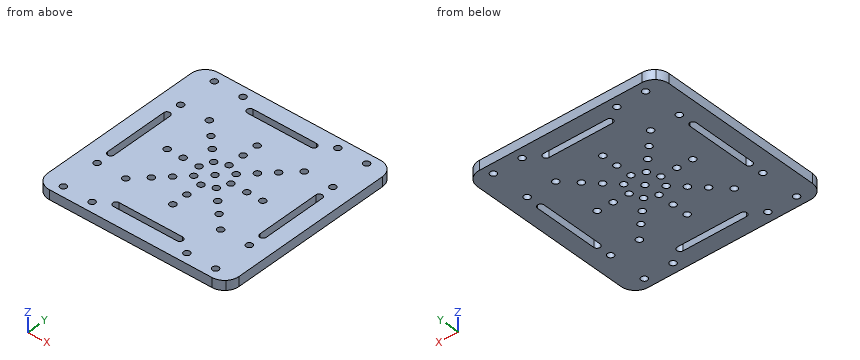
from build123d import *

# Parameters (mm, degrees)
F0_W     = 120
F0_H     = 6
F1_DEPTH = 120
F3_D     = 4
F3_DEPTH = 8
F3_TIP   = 1.2017212381
F4_DEPTH = 8
F5_DEPTH = 6


with BuildPart() as f1:
    # F0 (on Front) → F1 (new body)
    with BuildSketch(Plane.XZ):
        with Locations((60, 3)):
            Rectangle(F0_W, F0_H)
    extrude(amount=F1_DEPTH)

    # F3
    with Locations(Plane(origin=(0, 0, 0), x_dir=(1, 0, 0), z_dir=(0, 0, -1))):
        with Locations((12.2512626585, 113.7487373415), (12.2512626585, 89.7487373415), (30.2512626585, 89.7487373415), (30.2512626585, 113.7487373415), (89.7487373415, 113.7487373415), (89.7487373415, 89.7487373415), (107.7487373415, 89.7487373415), (107.7487373415, 113.7487373415), (107.7487373415, 30.2512626585), (89.7487373415, 30.2512626585), (89.7487373415, 6.2512626585), (107.7487373415, 6.2512626585), (30.2512626585, 6.2512626585), (12.2512626585, 30.2512626585), (30.2512626585, 30.2512626585), (12.2512626585, 6.2512626585), (38.7867965644, 38.7867965644), (45.8578643763, 45.8578643763), (30, 60), (40, 60), (45.8578643763, 74.1421356237), (38.7867965644, 81.2132034356), (60, 80), (60, 90), (81.2132034356, 81.2132034356), (74.1421356237, 74.1421356237), (80, 60), (90, 60), (81.2132034356, 38.7867965644), (74.1421356237, 45.8578643763), (60, 40), (60, 30), (52.9289321881, 67.0710678119), (60, 60), (50, 60), (52.9289321881, 52.9289321881), (60, 50), (67.0710678119, 52.9289321881), (70, 60), (67.0710678119, 67.0710678119), (60, 70)):
            Hole(F3_D / 2, depth=F3_DEPTH)
            with Locations((0, 0, -(F3_DEPTH + F3_TIP / 2))):  # 118° drill point
                Cone(0, F3_D / 2, F3_TIP, mode=Mode.SUBTRACT)

    # F2 (on Top) → F4 (cut)
    with BuildSketch(Plane.XY):
        with BuildLine():
            Line((10.2512626585, -40), (10.2512626585, -60))
            Line((10.2512626585, -60), (14.2512626585, -60))
            Line((14.2512626585, -60), (14.2512626585, -40))
            ThreePointArc((14.2512626585, -40), (12.2512626585, -38), (10.2512626585, -40))
        make_face()
        with BuildLine():
            Line((14.2512626585, -60), (10.2512626585, -60))
            Line((10.2512626585, -60), (10.2512626585, -80))
            ThreePointArc((10.2512626585, -80), (12.2512626585, -82), (14.2512626585, -80))
            Line((14.2512626585, -80), (14.2512626585, -60))
        make_face()
        with BuildLine():
            Line((60, -109.7487373415), (60, -105.7487373415))
            Line((60, -105.7487373415), (40, -105.7487373415))
            ThreePointArc((40, -105.7487373415), (38, -107.7487373415), (40, -109.7487373415))
            Line((40, -109.7487373415), (60, -109.7487373415))
        make_face()
        with BuildLine():
            Line((80, -105.7487373415), (60, -105.7487373415))
            Line((60, -105.7487373415), (60, -109.7487373415))
            Line((60, -109.7487373415), (80, -109.7487373415))
            ThreePointArc((80, -109.7487373415), (82, -107.7487373415), (80, -105.7487373415))
        make_face()
        with BuildLine():
            Line((105.7487373415, -40), (105.7487373415, -60))
            Line((105.7487373415, -60), (109.7487373415, -60))
            Line((109.7487373415, -60), (109.7487373415, -40))
            ThreePointArc((109.7487373415, -40), (107.7487373415, -38), (105.7487373415, -40))
        make_face()
        with BuildLine():
            Line((109.7487373415, -60), (105.7487373415, -60))
            Line((105.7487373415, -60), (105.7487373415, -80))
            ThreePointArc((105.7487373415, -80), (107.7487373415, -82), (109.7487373415, -80))
            Line((109.7487373415, -80), (109.7487373415, -60))
        make_face()
        with BuildLine():
            Line((40, -14.2512626585), (60, -14.2512626585))
            Line((60, -14.2512626585), (60, -10.2512626585))
            Line((60, -10.2512626585), (40, -10.2512626585))
            ThreePointArc((40, -10.2512626585), (38, -12.2512626585), (40, -14.2512626585))
        make_face()
        with BuildLine():
            Line((60, -10.2512626585), (60, -14.2512626585))
            Line((60, -14.2512626585), (80, -14.2512626585))
            ThreePointArc((80, -14.2512626585), (82, -12.2512626585), (80, -10.2512626585))
            Line((80, -10.2512626585), (60, -10.2512626585))
        make_face()
    extrude(amount=F4_DEPTH, mode=Mode.SUBTRACT)

    # F2 (on Top) → F5 (cut)
    with BuildSketch(Plane.XY):
        with BuildLine():
            Line((120, -120), (120, -111))
            ThreePointArc((120, -111), (119.3149157926, -114.4441508913), (117.3639610307, -117.3639610307))
            Line((117.3639610307, -117.3639610307), (120, -120))
        make_face()
        with BuildLine():
            ThreePointArc((117.3639610307, -117.3639610307), (114.4441508913, -119.3149157926), (111, -120))
            Line((111, -120), (120, -120))
            Line((120, -120), (117.3639610307, -117.3639610307))
        make_face()
        with BuildLine():
            Line((2.6360389693, -117.3639610307), (0, -120))
            Line((0, -120), (9, -120))
            ThreePointArc((9, -120), (5.5558491087, -119.3149157926), (2.6360389693, -117.3639610307))
        make_face()
        with BuildLine():
            ThreePointArc((2.6360389693, -117.3639610307), (0.6850842074, -114.4441508913), (0, -111))
            Line((0, -111), (0, -120))
            Line((0, -120), (2.6360389693, -117.3639610307))
        make_face()
        with BuildLine():
            ThreePointArc((117.3639610307, -2.6360389693), (119.3149157926, -5.5558491087), (120, -9))
            Line((120, -9), (120, 0))
            Line((120, 0), (117.3639610307, -2.6360389693))
        make_face()
        with BuildLine():
            Line((120, 0), (111, 0))
            ThreePointArc((111, 0), (114.4441508913, -0.6850842074), (117.3639610307, -2.6360389693))
            Line((117.3639610307, -2.6360389693), (120, 0))
        make_face()
        with BuildLine():
            Line((0, 0), (0, -9))
            ThreePointArc((0, -9), (0.6850842074, -5.5558491087), (2.6360389693, -2.6360389693))
            Line((2.6360389693, -2.6360389693), (0, 0))
        make_face()
        with BuildLine():
            Line((9, 0), (0, 0))
            Line((0, 0), (2.6360389693, -2.6360389693))
            ThreePointArc((2.6360389693, -2.6360389693), (5.5558491087, -0.6850842074), (9, 0))
        make_face()
    extrude(amount=F5_DEPTH, mode=Mode.SUBTRACT)


solid = f1.part
Part model, mm, in its own coordinate system. Round coordinates to 2 decimals unless told otherwise and drop trailing zeros. Write each loop counter-clockwise with the first axis right and the second up, starting at its lowest first coordinate (ties: lowest second). Pieces come first, ordered by that corner, then holes. Notation, with made-up numbers: M 76,84 L 130,84 A30 cw 130,113 Z; hole C 37,0.5 d11. An arc over 180 degrees is marked long. Return JSON: item names as keys, results as strings. Group by question number.
(1) Saw through at A-A on x = 107.5. Write the cut outline in (y, z).
(2) Drill centre lines: probe 1 along Y at (x, z) = (65, 2.1); probe 2 along X at (y, z) = (-30, 2.5); probe 3 along Y at (x, z) = (30, 0.8). Where is each one in solid material? Low to high.
(3) Saw through at B-B on z = 4.65. Count the separate pieces of the cut face and the enclosed holes in it, then the cut area to 3 significant figures.
Returned:
{
 "1": {"outline": "M -120,0 L -115.73,0 L -115.73,6 L -120,6 Z; M -111.76,0 L -91.73,0 L -91.73,6 L -111.76,6 Z; M -87.76,0 L -81.98,0 L -81.98,6 L -87.76,6 Z; M -38.02,0 L -32.24,0 L -32.24,6 L -38.02,6 Z; M -28.27,0 L -8.24,0 L -8.24,6 L -28.27,6 Z; M -4.27,0 L 0,0 L 0,6 L -4.27,6 Z"},
 "2": {"probe 1": "-120 to -109.75, -105.75 to -14.25, -10.25 to 0", "probe 2": "0 to 10.27, 14.24 to 28.27, 32.24 to 58, 62 to 87.76, 91.73 to 105.76, 109.73 to 120", "probe 3": "-120 to -115.73, -111.76 to -91.73, -87.76 to -62, -58 to -32.24, -28.27 to -8.24, -4.27 to 0"},
 "3": {"separate pieces": "1", "enclosed holes": "45", "area": "13,100 mm²"}
}
